```python
from build123d import *

# Parameters (mm, degrees)
AUFSATZ_LINEAR_AUSTRAGEN1_DEPTH      = 8
AUFSATZ_LINEAR_AUSTRAGEN2_DEPTH      = 91
SCHNITT_LINEAR_AUSTRAGEN1_DEPTH      = 105.959516136
SCHNITT_LINEAR_AUSTRAGEN1_DEPTH_BACK = 105.959516136


with BuildPart() as part:
    # Skizze1 → Rotation3 (revolve)
    with BuildSketch(Plane.XY, mode=Mode.PRIVATE) as rotation3_sk:
        with BuildLine():
            Line((-9.704368381, -98.133930518), (-9.932000587, -97.840841346))
            ThreePointArc((-9.932000587, -97.840841346), (-15.555484295, -87.430194788), (-17.5, -75.758691482))
            Line((-17.5, -75.758691482), (-17.5, -43.769743195))
            ThreePointArc((-17.5, -43.769743195), (-16.512197538, -35.394420898), (-13.60299869, -27.478718823))
            Line((-13.60299869, -27.478718823), (-12.198660374, -24.711337836))
            ThreePointArc((-12.198660374, -24.711337836), (-10.099873178, -17.28685515), (-10.967624651, -9.620378892))
            Line((-10.967624651, -9.620378892), (-13.60299869, -1.302019492))
            ThreePointArc((-13.60299869, -1.302019492), (-13.45654869, -0.409246029), (-12.649696941, 0))
            Line((-12.649696941, 0), (0, 0))
            Line((0, 0), (0, -102))
            Line((0, -102), (-1.80659044, -102))
            ThreePointArc((-1.80659044, -102), (-6.203219536, -100.981628616), (-9.704368381, -98.133930518))
        make_face()
    revolve(rotation3_sk.sketch.rotate(Axis((0, 79.626152289, 0), (0, -1, 0)), 270), axis=Axis((0, 79.626152289, 0), (0, -1, 0)))

    # Skizze2 → Aufsatz-Linear austragen1 (add)
    with BuildSketch(Plane(origin=(0, 0, 0), x_dir=(1, 0, 0), z_dir=(0, 1, 0))):
        Polygon((-4, -2.309401077), (0, -4.618802154), (4, -2.309401077), (4, 2.309401077), (0, 4.618802154), (-4, 2.309401077), align=None)
    extrude(amount=AUFSATZ_LINEAR_AUSTRAGEN1_DEPTH)

    # Skizze3 → Aufsatz-Linear austragen2 (add)
    with BuildSketch(Plane(origin=(0, 8, 0), x_dir=(1, 0, 0), z_dir=(0, 1, 0))):
        Polygon((-3.25, -1.876388375), (0, -3.75277675), (3.25, -1.876388375), (3.25, 1.876388375), (0, 3.75277675), (-3.25, 1.876388375), align=None)
    extrude(amount=AUFSATZ_LINEAR_AUSTRAGEN2_DEPTH)

    # Skizze4 → Schnitt-Linear austragen1 (cut, two sides: drawn at the far end of the back side and taken through both)
    with BuildSketch(Plane(origin=(0, 0, 0), x_dir=(0, 0, -1), z_dir=(1, 0, 0)).offset(-SCHNITT_LINEAR_AUSTRAGEN1_DEPTH_BACK)):
        Polygon((-0.7, 99), (-3.75277675, 77), (-3.75277675, 99), align=None)
        Polygon((0.7, 99), (3.75277675, 77), (3.75277675, 99), align=None)
    extrude(amount=SCHNITT_LINEAR_AUSTRAGEN1_DEPTH + SCHNITT_LINEAR_AUSTRAGEN1_DEPTH_BACK, mode=Mode.SUBTRACT)


solid = part.part
```
Input: part model. Units: mm. Frame: model coordinates. A direction names the side the tool comes from. Round coordinates to 2 decimals unless told otherwise and drop trailing zeros. Loops run counter-clockwise (first coordinate to the right, second up) from the corner with the lowest first, then second, coordinate; pieces in that order, holes last. Notation, with made-up numbers: (62.25, -4) -> (111.25, -4) arc R31 ccw to (111.25, 23) -> close; hole circle Ø2 at (60.25, 79.25). An arc over 180 degrees is marked (long way). Use one line per item in the form item = value. Start each with the question number.
Item 1: Section query B-B on y = -58. Return the cut outline in (x, z).
Item 2: Section query A-A on y = 51. Return the cut outline in (x, z), then the cut area to 3 significant figures.
Item 3: Contact query for flat-ended pins moving along their axis: pin 1 Ø8 at (y, z) = (14, 1) entering from -X; pin 2 Ø1 at (x, z) = (-8, -8.5) entering from -Y; pin 3 Ø10 at (y, z) = (52, 7.5) entering from -X. Output: stop coordinate, or through.
Item 4: Material intervals for L1, parallel to Z at x = -8, y = -4; L2, parallel to Z at x = -11, y = -57.5; L3, parallel to X at y = -57.5, z = -1, sorted ascending. Write a range as from..to.
Item 5: Set-up query: faces 1 (the face through (3.25, 53, 0)), 2 (the face through (-4, 4, 0)), 3 (the face through (1.65, 48.68, -2.8)). Return all of +Z, -Z, +X, -X, +Y, -Y with unobstructed straight access to the full face (end or side cutting, diameter ignored); none if empty.
Ans:
q1.outline = circle Ø35 at (0, 0)
q2.outline = (-3.25, -1.88) -> (0, -3.75) -> (3.25, -1.88) -> (3.25, 1.88) -> (0, 3.75) -> (-3.25, 1.88) -> close
q2.area = 36.6 mm^2
q3.pin_1 = -3.25
q3.pin_2 = -96.14
q3.pin_3 = -2.17
q4.L1 = -9.93..9.93
q4.L2 = -13.61..13.61
q4.L3 = -17.47..17.47
q5.face_1 = +Z, -Z, +X, +Y
q5.face_2 = +Z, -Z, -X, +Y
q5.face_3 = -Z, +X, +Y
